For this review, use the dimensioned drawing (mm, ordinates from the lowest corner) and the shaded views. Give positions to 0.01 mm unless a question says otherwise; leave off trailing zeros. Order: outer loops, then holes, each group sorted by start corner. A loop starts at its lowest first (then second) coordinate and runs counter-clockwise, first axis right, second up. Notation, with made-up numbers: (61.25, 58) -> (99.25, 58) arc R6 cw to (99.25, 68) -> close; hole circle Ø9 at (17.5, -37). An arc over 180 degrees is marked (long way). One line per item, written item: value. Start each with the question number.
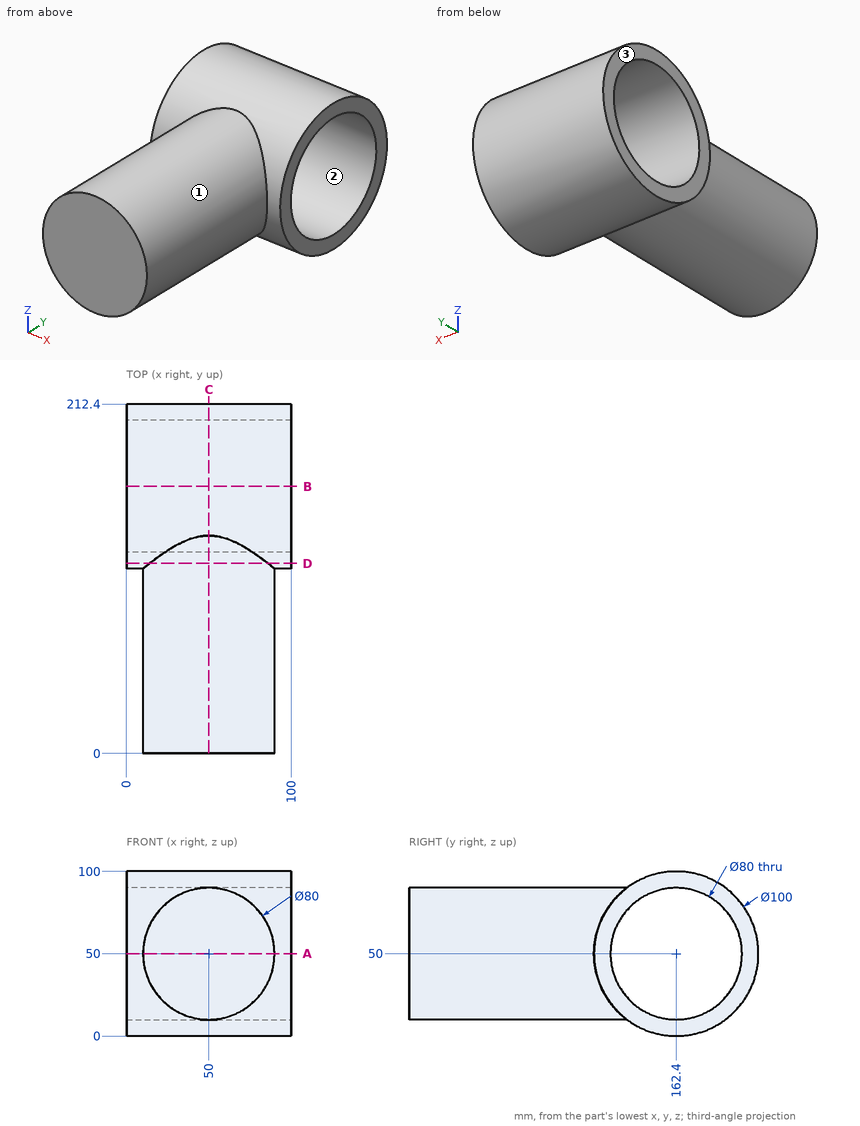
Q1. For pin 1 Ø3 at (x, y) = (65.5, 77) entering from +Z; pin 2 Ø5 at (x, z) = (23.5, 89) entering from -Y; pin 3 Ø8 at (y, z) = (41.5, 27.5) entering from -X, all flat-tipped, find the tip position at first contact; note any pin that passes through.
Q2. For line 1 along Y through (x, z) = (40, 50); line 2 along Z through (x, y) = (36, 164); line 3 along Y through (x, z) = (75, 23.5), list the stretches that pass through material, from the lowest coordinate up.
Q3. Take a section at B-B (y = 162.4). State the section outline as (x, z) points, and give its area (3 significant figures).
Q4. Take a section at C-C (x = 50). State the section outline as (y, z) points, and give its area (3 significant figures).
Q5. Take a section at A-A (z = 50). State the section outline as (x, y) points, and give its area (3 significant figures).
Q6. Take a section at D-D (y = 115.5). State the section outline as (x, z) points, and give its area (3 significant figures).
Q7. Mouldability with a two-part tool opening along Z and no side actions: class the marked faces 1, 2 and 3 as pulls with the +Z half, pulls with the -Z half, needs draft (parallel to the pull), parting line crosses it, or undercut.
Answers below:
1. pin 1: stops at z = 87.47
1. pin 2: stops at y = 128.23
1. pin 3: stops at x = 14.54
2. line 1: y = 0 to 122.4, 202.4 to 212.4
2. line 2: z = 0.03 to 10.03, 89.97 to 99.97
2. line 3: y = 0 to 132.44, 192.36 to 204.8
3. outline: (0, 0) -> (100, 0) -> (100, 10) -> (0, 10) -> close; (0, 90) -> (100, 90) -> (100, 100) -> (0, 100) -> close
3. area: 2,000 mm²
4. outline: (0, 10) -> (132.4, 10) arc R50 ccw (long way) to (132.4, 90) -> (0, 90) -> close; hole circle Ø80 at (162.4, 50)
4. area: 12,300 mm²
5. outline: (0, 112.4) -> (10, 112.4) -> (10, 0) -> (90, 0) -> (90, 112.4) -> (100, 112.4) -> (100, 122.4) -> (0, 122.4) -> close; (0, 202.4) -> (100, 202.4) -> (100, 212.4) -> (0, 212.4) -> close
5. area: 11,000 mm²
6. outline: (0, 32.67) -> (13.95, 32.67) arc R40 ccw to (86.05, 32.67) -> (100, 32.67) -> (100, 67.33) -> (86.05, 67.33) arc R40 ccw to (13.95, 67.33) -> (0, 67.33) -> close
6. area: 5,810 mm²
7. face 1: parting line crosses it
7. face 2: undercut
7. face 3: needs draft
